from build123d import *

# Parameters (mm, degrees)
BOSS_EXTRUDE2_START = 20
SKETCH3_R           = 70
SKETCH3_R_2         = 40
BOSS_EXTRUDE2_DEPTH = 20
SKETCH4_R           = 8
BOSS_EXTRUDE3_DEPTH = 80


with BuildPart() as part:
    # Sketch2 → Revolve1 (revolve)
    with BuildSketch(Plane.YZ):
        with BuildLine():
            Line((0, 0), (0, 70))
            ThreePointArc((0, 70), (25, 95), (50, 70))
            Line((50, 70), (40, 70))
            Line((40, 70), (40, 56))
            Line((40, 56), (50, 56))
            Line((50, 56), (50, 0))
            Line((50, 0), (0, 0))
        make_face()
    revolve(axis=Axis((0, 50, 0), (0, -1, 0)))

    # Sketch3 → Boss-Extrude2 (add)
    with BuildSketch(Plane.XZ.offset(BOSS_EXTRUDE2_START)):
        with Locations(Location((0, 0, 0), (0, 0, 90))):
            Circle(SKETCH3_R)
        with Locations(Location((0, 0, 0), (0, 0, 270))):
            Circle(SKETCH3_R_2, mode=Mode.SUBTRACT)
    extrude(amount=-BOSS_EXTRUDE2_DEPTH)

    # Sketch4 → Boss-Extrude3 (add)
    with BuildSketch(Plane.XZ):
        with Locations(Location((0, 0, 0), (0, 0, 270))):
            Circle(SKETCH4_R)
    extrude(amount=BOSS_EXTRUDE3_DEPTH)


solid = part.part
Work out the finished part from the listing and answer in its coordinate system (mm). A direction names the side the tool comes from. Round coordinates to 2 decimals unless told otherwise and drop trailing zeros. Write each loop counter-clockwise with the first axis right and the second up, starting at its lowest first coordinate (ties: lowest second). Pieces come first, ordered by that corner, then holes. Notation, with made-up numbers: (64.25, 73) - (85.25, 73) arc R19 ccw to (85.25, 77) - close; hole circle Ø8 at (67, -35). An arc over 180 degrees is marked (long way). Answer in a Markdown table with one row per item. Add a question column.
1. A cutting plane is placed at D-D, the plane y = 28.5. Determine the outline of the cut face in (x, z), and give its area (3 significant figures).
2. The mould has two halves that part along Z. Classify faces 1 (the cylindrical face through (42.594, 44.93, -55.55)), 2 (the flat face through (0, -80, 0)), 3 (the cylindrical face through (42.594, -10.14, -55.55)): +Z half, -Z half, draft (parallel to the pull), parting line (faces both ways), or undercut.
3. For faces 4 (the flat face through (-1, 50, -1)), 5 (the flat face through (-0.6, 0, -8.3)), 6 (the cylindrical face through (21.45, 45.07, 51.73)), determine the directions among +Z, -Z, +X, -X, +Y, -Y from which every point of the face is accessible in a straight line to the end or side of a thin tool.
4. Given pin 1 (3 mm diameter, centred on x = 67, y = 31, fed in from +Z); pin 2 (12 mm diameter, centred on x = -63, y = 1, fed in from +Z); pin 3 (12 mm diameter, centred on x = -62, z = 39, fed in from -Y), each flat-ended and moving along its own axis, determine where each tip first touches the part or whether it passes through.
5. A cutting plane is placed at B-B, the plane z = 0. Determine the outline of the cut face in (x, y), and give its area (3 significant figures).
6. A cutting plane is placed at C-C, the plane y = -25. Determine the outline of the cut face in (x, z).
7. Find the intervals of material crossed by line 1 along Z through (x, y) = (0, 43); line 2 along X through (y, z) = (-1, 2.5); line 3 along Z through (x, y) = (0, 44.5), in increasing order. Write a range as from..to.
8. A cutting plane is placed at A-A, the plane x = 0. Determine the outline of the cut face in (y, z).
Worked out:
| question | item | result |
|---|---|---|
| 1 | outline | circle Ø189.51 at (0, 0) |
| 1 | area | 28,200 mm^2 |
| 2 | face 1 | undercut |
| 2 | face 2 | draft |
| 2 | face 3 | parting line |
| 3 | face 4 | +Z, -Z, +X, -X, +Y |
| 3 | face 5 | -Y |
| 3 | face 6 | +Y |
| 4 | pin 1 | z = 67.88 |
| 4 | pin 2 | z = 62.27 |
| 4 | pin 3 | y = -20 |
| 5 | outline | (-70, -20) - (-40, -20) - (-40, 0) - (-8, 0) - (-8, -80) - (8, -80) - (8, 0) - (40, 0) - (40, -20) - (70, -20) - (70, 0) arc R25 ccw to (70, 50) - (70, 40) - (56, 40) - (56, 50) - (-56, 50) - (-56, 40) - (-70, 40) - (-70, 50) arc R25 ccw to (-70, 0) - close |
| 5 | area | 11,200 mm^2 |
| 6 | outline | circle Ø16 at (0, 0) |
| 7 | line 1 | -87.35..-70, -56..56, 70..87.35 |
| 7 | line 2 | -69.96..-39.92, -7.6..7.6, 39.92..69.96 |
| 7 | line 3 | -85.64..-70, -56..56, 70..85.64 |
| 8 | outline | (-80, -8) - (0, -8) - (0, -40) - (-20, -40) - (-20, -70) - (0, -70) arc R25 ccw to (50, -70) - (40, -70) - (40, -56) - (50, -56) - (50, 56) - (40, 56) - (40, 70) - (50, 70) arc R25 ccw to (0, 70) - (-20, 70) - (-20, 40) - (0, 40) - (0, 8) - (-80, 8) - close |
